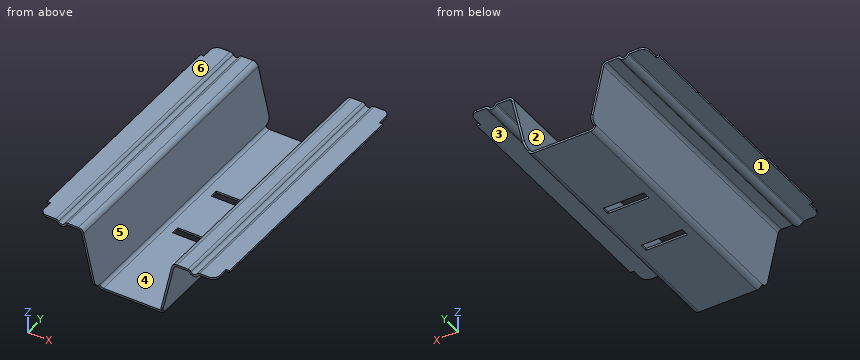
```python
from build123d import *

# Parameters (mm, degrees)
EXTRUDE_THIN1_DEPTH = 20.5
EXTRUDE1_DEPTH      = 41
EXTRUDE2_DEPTH      = 1
FILLET1_R           = 1
EXTRUDE3_DEPTH      = 1
FILLET2_R           = 1
SKETCH5_W           = 6.1
SKETCH5_H           = 1.22
EXTRUDE4_DEPTH      = 45.5


with BuildPart() as part:
    # Sketch1 → Extrude-Thin1 (new, symmetric)
    with BuildSketch(Plane(origin=(0, 0, 0), x_dir=(1, 0, 0), z_dir=(0, 1, 0))):
        with BuildLine():
            Line((13.5, 0), (10.666025404, 0))
            ThreePointArc((10.666025404, 0), (10.416025404, 0.066987298), (10.233012702, 0.25))
            ThreePointArc((10.233012702, 0.25), (9.8, 0.5), (9.366987298, 0.25))
            ThreePointArc((9.366987298, 0.25), (9.183974596, 0.066987298), (8.933974596, 0))
            Line((8.933974596, 0), (7.3, 0))
            ThreePointArc((7.3, 0), (6.800019439, 0.175484637), (6.519386146, 0.624951403))
            Line((6.519386146, 0.624951403), (4.737883659, 8.569405373))
            ThreePointArc((4.737883659, 8.569405373), (4.56248785, 8.850322102), (4.25, 8.96))
            Line((4.25, 8.96), (-4.25, 8.96))
            ThreePointArc((-4.25, 8.96), (-4.56248785, 8.850322102), (-4.737883659, 8.569405373))
            Line((-4.737883659, 8.569405373), (-6.519386146, 0.624951403))
            ThreePointArc((-6.519386146, 0.624951403), (-6.800019439, 0.175484637), (-7.3, 0))
            Line((-7.3, 0), (-8.933974596, 0))
            ThreePointArc((-8.933974596, 0), (-9.183974596, 0.066987298), (-9.366987298, 0.25))
            ThreePointArc((-9.366987298, 0.25), (-9.8, 0.5), (-10.233012702, 0.25))
            ThreePointArc((-10.233012702, 0.25), (-10.416025404, 0.066987298), (-10.666025404, 0))
            Line((-10.666025404, 0), (-13.5, 0))
            Line((-13.5, 0), (-13.5, 0.3))
            Line((-13.5, 0.3), (-10.666025404, 0.3))
            ThreePointArc((-10.666025404, 0.3), (-10.566025404, 0.326794919), (-10.492820323, 0.4))
            ThreePointArc((-10.492820323, 0.4), (-9.8, 0.8), (-9.107179677, 0.4))
            ThreePointArc((-9.107179677, 0.4), (-9.033974596, 0.326794919), (-8.933974596, 0.3))
            Line((-8.933974596, 0.3), (-7.3, 0.3))
            ThreePointArc((-7.3, 0.3), (-6.98751215, 0.409677898), (-6.812116341, 0.690594627))
            Line((-6.812116341, 0.690594627), (-5.030613854, 8.635048597))
            ThreePointArc((-5.030613854, 8.635048597), (-4.749980561, 9.084515363), (-4.25, 9.26))
            Line((-4.25, 9.26), (4.25, 9.26))
            ThreePointArc((4.25, 9.26), (4.749980561, 9.084515363), (5.030613854, 8.635048597))
            Line((5.030613854, 8.635048597), (6.812116341, 0.690594627))
            ThreePointArc((6.812116341, 0.690594627), (6.98751215, 0.409677898), (7.3, 0.3))
            Line((7.3, 0.3), (8.933974596, 0.3))
            ThreePointArc((8.933974596, 0.3), (9.033974596, 0.326794919), (9.107179677, 0.4))
            ThreePointArc((9.107179677, 0.4), (9.8, 0.8), (10.492820323, 0.4))
            ThreePointArc((10.492820323, 0.4), (10.566025404, 0.326794919), (10.666025404, 0.3))
            Line((10.666025404, 0.3), (13.5, 0.3))
            Line((13.5, 0.3), (13.5, 0))
        make_face()
    extrude(amount=EXTRUDE_THIN1_DEPTH, both=True)

    # Sketch2 → Extrude1 (cut)
    with BuildSketch(Plane.XY):
        with BuildLine():
            Line((-13.5, 18), (-13, 18))
            Line((-13, 18), (-13, 19.5))
            ThreePointArc((-13, 19.5), (-12.707106781, 20.207106781), (-12, 20.5))
            Line((-12, 20.5), (0, 20.5))
            Line((0, 20.5), (12, 20.5))
            ThreePointArc((12, 20.5), (12.707106781, 20.207106781), (13, 19.5))
            Line((13, 19.5), (13, 18))
            Line((13, 18), (13.5, 18))
            Line((13.5, 18), (13.5, 21.5))
            Line((13.5, 21.5), (-13.5, 21.5))
            Line((-13.5, 21.5), (-13.5, 18))
        make_face()
        with BuildLine():
            Line((-13.5, -18), (-13, -18))
            Line((-13, -18), (-13, -19.5))
            ThreePointArc((-13, -19.5), (-12.707106781, -20.207106781), (-12, -20.5))
            Line((-12, -20.5), (12, -20.5))
            ThreePointArc((12, -20.5), (12.707106781, -20.207106781), (13, -19.5))
            Line((13, -19.5), (13, -18))
            Line((13, -18), (13.5, -18))
            Line((13.5, -18), (13.5, -21.5))
            Line((13.5, -21.5), (-13.5, -21.5))
            Line((-13.5, -21.5), (-13.5, -18))
        make_face()
    extrude(amount=-EXTRUDE1_DEPTH, mode=Mode.SUBTRACT)

    # Sketch3 → Extrude2 (cut)
    with BuildSketch(Plane(origin=(0, 20.5, 0), x_dir=(1, 0, 0), z_dir=(0, 1, 0))):
        Polygon((-5.030613854, 8.635048597), (-4.737883659, 8.569405373), (4.737883659, 8.569405373), (5.030613854, 8.635048597), (5.030613854, 9.569405373), (-5.030613854, 9.569405373), align=None)
    extrude(amount=-EXTRUDE2_DEPTH, mode=Mode.SUBTRACT)

    # Fillet1
    fillet1_edges = [part.edges().sort_by_distance(p)[0] for p in [
        (-4.884248756, 20.5, -8.602226985),
        (4.884248756, 20.5, -8.602226985),
    ]]
    fillet(fillet1_edges, radius=FILLET1_R - 0.0001)  # a hair under: the kernel refuses the full size

    # Sketch4 → Extrude3 (cut)
    with BuildSketch(Plane.XZ.offset(20.5)):
        Polygon((-4.737883659, -8.569405373), (-5.030613854, -8.635048597), (-5.030613854, -10.26), (5.030613854, -10.26), (5.030613854, -8.635048597), (4.737883659, -8.569405373), align=None)
    extrude(amount=-EXTRUDE3_DEPTH, mode=Mode.SUBTRACT)

    # Fillet2
    fillet2_edges = [part.edges().sort_by_distance(p)[0] for p in [
        (4.884248756, -20.5, -8.602226985),
        (-4.884248756, -20.5, -8.602226985),
    ]]
    fillet(fillet2_edges, radius=FILLET2_R - 0.0001)  # a hair under: the kernel refuses the full size

    # Sketch5 → Extrude4 (cut)
    with BuildSketch(Plane.XY):
        with Locations((0, 4.51)):
            Rectangle(SKETCH5_W, SKETCH5_H)
        with Locations((0, -4.51)):
            Rectangle(SKETCH5_W, SKETCH5_H)
    extrude(amount=-EXTRUDE4_DEPTH, mode=Mode.SUBTRACT)


solid = part.part
```
Verification items for the finished model (mm, model axes). Face numbers are marked on the shaded views. A direction names the side the tool comes from. Coordinates: 2 decimals unless noted, no trailing zeros. Write each loop counter-clockwise with the first axis right and the second up, starting at its lowest first coordinate (ties: lowest second). Pieces come first, ordered by that corner, then holes. Notation, with made-up numbers: M 87,58.5 L 103,58.5 A25 cw 103,80.5 Z; hole C -15,-33 d8. An arc over 180 degrees is marked long. Answer as a JSON object with one key per item and string values. Group by question number.
(1) Gauge pin test, flat ends, axial feed: pin 1 (5 mm diameter, centred on y = 9, z = -6, fed in from -X); pin 2 (5 mm diameter, centred on x = -5.5, z = -4.5, fed in from +Y); pin 3 (2.5 mm diameter, centred on x = -12, y = -4, fed in from -Z); pin 4 (0.8 mm diameter, centred on x = -2, z = -9, fed in from +Y). Record the tip position at first contact, or that the pin passes through.
(2) Material ranges on line 1 (Z direction, x = -12, y = 2.5); line 2 (X direction, y = -5, z = -1.5); line 3 (X direction, y = -14.5, z = -6), recorded low to high.
(3) Cross-section at A-A, the plane z = -6.5. Record the cut outline in (x, y), and give its area (3 significant figures).
(4) Release check for a two-part mould opening along X. For the marked faces 4, 5 and 6 record: +X half, -X half, draft (parallel to the pull), parting line (faces both ways), or undercut.
(5) Tool access check on the marked faces 1, 2 and 3. Record the directions out of +Z, -Z, +X, -X, +Y, -Y that give a thin tool (end or side, any length) a straight path to the whole face; none if there is none.
(6) Cross-section at B-B, the plane x = 8. Record the cut outline in (y, z).
Reply:
{
 "1": {"pin 1": "x = -6.18", "pin 2": "y = 20.5", "pin 3": "z = -0.3", "pin 4": "y = 19.5"},
 "2": {"line 1": "-0.3 to 0", "line 2": "-6.63 to -6.32, 6.32 to 6.63", "line 3": "-5.62 to -5.31, 5.31 to 5.62"},
 "3": {"outline": "M -5.51,-20.5 L -5.2,-20.5 L -5.2,20.5 L -5.51,20.5 Z; M 5.2,-20.5 L 5.51,-20.5 L 5.51,20.5 L 5.2,20.5 Z", "area": "25.2 mm²"},
 "4": {"face 4": "undercut", "face 5": "undercut", "face 6": "draft"},
 "5": {"face 1": "-Z, -X, +Y, -Y", "face 2": "+Z, +Y, -Y", "face 3": "-Z, +X, +Y, -Y"},
 "6": {"outline": "M -20.5,-0.3 L 20.5,-0.3 L 20.5,0 L -20.5,0 Z"}
}
